```python
from build123d import *

# Parameters (mm, degrees)
BOSS_EXTRUDE33_DEPTH = 5
BOSS_EXTRUDE34_START = 5
BOSS_EXTRUDE34_DEPTH = 1
BOSS_EXTRUDE35_START = -7
BOSS_EXTRUDE35_DEPTH = 7
CUT_EXTRUDE2_DEPTH   = 2


with BuildPart() as part:
    # lid → Boss-Extrude33 (new body)
    with BuildSketch(Plane(origin=(0, 0, 0), x_dir=(1, 0, 0), z_dir=(0, 1, 0))):
        with BuildLine():
            Line((11.25, 15), (10.5, 15))
            Line((10.5, 15), (10.5, -7.65))
            ThreePointArc((10.5, -7.65), (10.353553391, -8.003553391), (10, -8.15))
            Line((10, -8.15), (-10, -8.15))
            ThreePointArc((-10, -8.15), (-10.353553391, -8.003553391), (-10.5, -7.65))
            Line((-10.5, -7.65), (-10.5, 15))
            Line((-10.5, 15), (-11.25, 15))
            Line((-11.25, 15), (-11.25, -7.9))
            ThreePointArc((-11.25, -7.9), (-10.957106781, -8.607106781), (-10.25, -8.9))
            Line((-10.25, -8.9), (10.25, -8.9))
            ThreePointArc((10.25, -8.9), (10.957106781, -8.607106781), (11.25, -7.9))
            Line((11.25, -7.9), (11.25, 15))
        make_face()
        with BuildLine():
            Line((9.25, 21.75), (9.25, 15))
            Line((9.25, 15), (10.5, 15))
            Line((10.5, 15), (11.25, 15))
            Line((11.25, 15), (11.25, 22))
            ThreePointArc((11.25, 22), (10.957106781, 22.707106781), (10.25, 23))
            Line((10.25, 23), (-10.25, 23))
            ThreePointArc((-10.25, 23), (-10.957106781, 22.707106781), (-11.25, 22))
            Line((-11.25, 22), (-11.25, 15))
            Line((-11.25, 15), (-10.5, 15))
            Line((-10.5, 15), (-9.25, 15))
            Line((-9.25, 15), (-9.25, 21.75))
            ThreePointArc((-9.25, 21.75), (-9.103553391, 22.103553391), (-8.75, 22.25))
            Line((-8.75, 22.25), (8.75, 22.25))
            ThreePointArc((8.75, 22.25), (9.103553391, 22.103553391), (9.25, 21.75))
        make_face()
    extrude(amount=BOSS_EXTRUDE33_DEPTH)

    # lid_5 → Boss-Extrude34 (add)
    with BuildSketch(Plane(origin=(0, 0, 0), x_dir=(1, 0, 0), z_dir=(0, 1, 0)).offset(BOSS_EXTRUDE34_START)):
        with BuildLine():
            ThreePointArc((11.25, 22), (10.957106781, 22.707106781), (10.25, 23))
            Line((10.25, 23), (-10.25, 23))
            ThreePointArc((-10.25, 23), (-10.957106781, 22.707106781), (-11.25, 22))
            Line((-11.25, 22), (-11.25, -7.9))
            ThreePointArc((-11.25, -7.9), (-10.957106781, -8.607106781), (-10.25, -8.9))
            Line((-10.25, -8.9), (10.25, -8.9))
            ThreePointArc((10.25, -8.9), (10.957106781, -8.607106781), (11.25, -7.9))
            Line((11.25, -7.9), (11.25, 22))
        make_face()
    extrude(amount=BOSS_EXTRUDE34_DEPTH)

    # lid_6 → Boss-Extrude35 (add)
    with BuildSketch(Plane(origin=(0, 0, 0), x_dir=(1, 0, 0), z_dir=(0, 1, 0)).offset(BOSS_EXTRUDE35_START)):
        with BuildLine():
            Line((9.25, 21.75), (9.25, 15))
            Line((9.25, 15), (10.5, 15))
            Line((10.5, 15), (11.25, 15))
            Line((11.25, 15), (11.25, 22))
            ThreePointArc((11.25, 22), (10.957106781, 22.707106781), (10.25, 23))
            Line((10.25, 23), (-10.25, 23))
            ThreePointArc((-10.25, 23), (-10.957106781, 22.707106781), (-11.25, 22))
            Line((-11.25, 22), (-11.25, 15))
            Line((-11.25, 15), (-10.5, 15))
            Line((-10.5, 15), (-9.25, 15))
            Line((-9.25, 15), (-9.25, 21.75))
            ThreePointArc((-9.25, 21.75), (-9.103553391, 22.103553391), (-8.75, 22.25))
            Line((-8.75, 22.25), (8.75, 22.25))
            ThreePointArc((8.75, 22.25), (9.103553391, 22.103553391), (9.25, 21.75))
        make_face()
    extrude(amount=BOSS_EXTRUDE35_DEPTH)

    # Sketch20 → Cut-Extrude2 (cut)
    with BuildSketch(Plane(origin=(0, 6, 0), x_dir=(1, 0, 0), z_dir=(0, 1, 0))):
        with BuildLine():
            Line((-7.672345443, -2.966739157), (7.39782559, -2.966739157))
            ThreePointArc((7.39782559, -2.966739157), (8.993011438, -4.561925004), (7.39782559, -6.157110852))
            Line((7.39782559, -6.157110852), (-7.672345443, -6.157110852))
            ThreePointArc((-7.672345443, -6.157110852), (-9.26753129, -4.561925004), (-7.672345443, -2.966739157))
        make_face()
    extrude(amount=-CUT_EXTRUDE2_DEPTH, mode=Mode.SUBTRACT)


solid = part.part
```
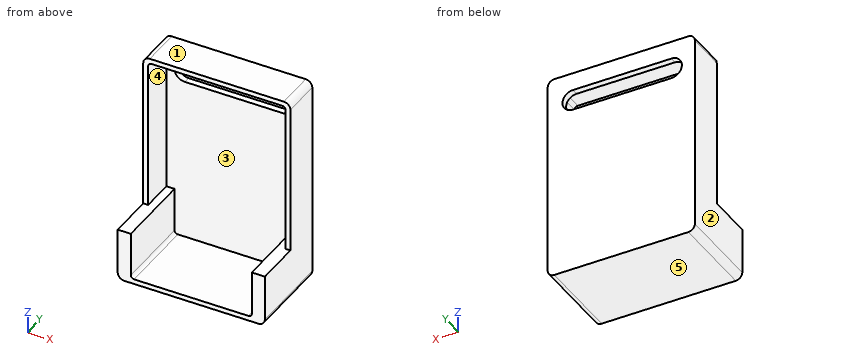
Model file for the job. Use its own axes, mm. Face numbers are marked on the shaded views. A direction names the side the tool comes from. Coordinates: 2 decimals unless noted, no trailing zeros. Order: outer loops, then holes, each group sorted by start corner. A loop starts at its lowest first (then second) coordinate and runs counter-clockwise, first axis right, second up. Notation, with made-up numbers: (-34.5, 29.5) - (15.5, 29.5) arc R25 ccw to (15.5, 55.5) - close; hole circle Ø2 at (51, 1.5). An arc over 180 degrees is marked (long way). Return JSON: item names as keys, results as strings. Group by question number.
1) Saw through at D-D, the plane z = 3.5. Write the cut outline in (x, y).
2) Mould opens along Z. For the marked faces 1, 2 and 3 say: released by +Z, released by -Z, zero draft, split by the parting line, or undercut.
3) Saw through at A-A, the plane x = 2.5. Write the cut outline in (y, z).
4) Probe line 1 (X direction, y = 2.25, z = -14.5); line 2 (X direction, y = -4.5, z = -19); line 3 (Z direction, x = -2, y = 4). List the from-to ranges inside material, lowest first. Write a range as from..to.
5) Tool access for the marked faces 4 and 5: list every direction of +Z, -Z, +X, -X, +Y, -Y with a clear straight run to the whole face (end or side of a thin tool).
6) Saw through at C-C, the plane z = -16. Write the cut outline in (x, y).
7) Flat gauge pins, fed straight in: P1, Ø2, axis at x = -7.5, z = 4, coming from the +Y side; P2, Ø1.6, axis at x = 10.5, y = -1.5, coming from the +Z side; P3, Ø10.5, axis at x = 1.5, z = -6, coming from the -Y side. Where does each tip first touch, or does it go through?
8) Saw through at B-B, the plane y = 4.5. Write the cut outline in (x, z), plus the area to 3 significant figures.
Values found:
{
 "1": {"outline": "(-11.25, 0) - (-10.5, 0) - (-10.5, 5) - (-8.86, 5) - (-8.86, 6) - (-11.25, 6) - close; (8.59, 5) - (10.5, 5) - (10.5, 0) - (11.25, 0) - (11.25, 6) - (8.59, 6) - close"},
 "2": {"face 1": "released by +Z", "face 2": "zero draft", "face 3": "undercut"},
 "3": {"outline": "(-7, -23) - (6, -23) - (6, 2.97) - (5, 2.97) - (5, -22.25) - (-7, -22.25) - close; (0, 8.15) - (5, 8.15) - (5, 6.16) - (6, 6.16) - (6, 8.9) - (0, 8.9) - close"},
 "4": {"line 1": "x = -11.25..-10.5, 10.5..11.25", "line 2": "x = -11.25..-9.25, 9.25..11.25", "line 3": "z = -23..-22.25, 8.15..8.9"},
 "5": {"face 4": "-Y", "face 5": "-Z, +X, -X, +Y, -Y"},
 "6": {"outline": "(-11.25, -7) - (-9.25, -7) - (-9.25, 5) - (9.25, 5) - (9.25, -7) - (11.25, -7) - (11.25, 6) - (-11.25, 6) - close"},
 "7": {"P1": "passes through", "P2": "stops at z = -15", "P3": "stops at y = 5"},
 "8": {"outline": "(-11.25, -22) arc R1 ccw to (-10.25, -23) - (10.25, -23) arc R1 ccw to (11.25, -22) - (11.25, 7.9) arc R1 ccw to (10.25, 8.9) - (-10.25, 8.9) arc R1 ccw to (-11.25, 7.9) - close; hole (-10.5, -15) - (-9.25, -15) - (-9.25, -21.75) arc R0.5 ccw to (-8.75, -22.25) - (8.75, -22.25) arc R0.5 ccw to (9.25, -21.75) - (9.25, -15) - (10.5, -15) - (10.5, 7.65) arc R0.5 ccw to (10, 8.15) - (-10, 8.15) arc R0.5 ccw to (-10.5, 7.65) - close", "area": "96.8 mm²"}
}
